from build123d import *

# Parameters (mm, degrees)
BOSS_EXTRUDE1_DEPTH = 10
SKETCH4_W           = 10
SKETCH4_H           = 2.5
SKETCH5_R           = 2.5
BOSS_EXTRUDE2_DEPTH = 5


with BuildPart() as part:
    # Sketch2 → Boss-Extrude1 (new body)
    with BuildSketch(Plane.XY):
        with BuildLine():
            Line((20, 0), (-20, 0))
            ThreePointArc((-20, 0), (0, 20), (20, 0))
        make_face()
    extrude(amount=BOSS_EXTRUDE1_DEPTH)

    # Sketch4 → Cut-Revolve1 (revolve, cut)
    with BuildSketch(Plane(origin=(0, 0, 0), x_dir=(0, 0, -1), z_dir=(1, 0, 0))):
        with Locations((-5, 1.25)):
            Rectangle(SKETCH4_W, SKETCH4_H)
    revolve(axis=Axis((0, 0, 17.133909945), (0, 0, -1)), mode=Mode.SUBTRACT)

    # Sketch5 → Boss-Extrude2 (add)
    with BuildSketch(Plane.XZ):
        with Locations((-15, 5)):
            Circle(SKETCH5_R)
        with Locations((15, 5)):
            Circle(SKETCH5_R)
    extrude(amount=BOSS_EXTRUDE2_DEPTH)


solid = part.part
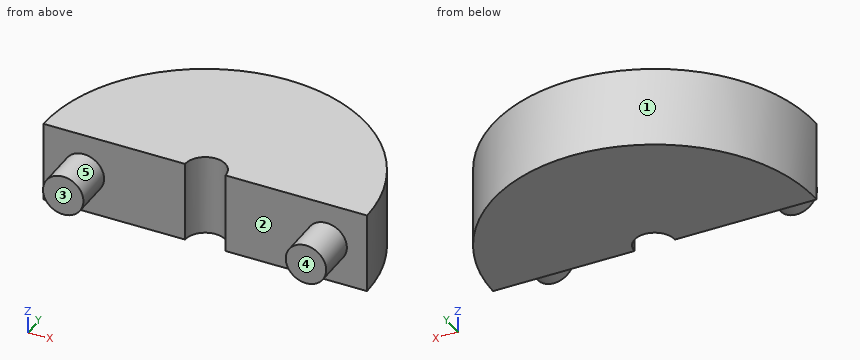
The listing builds one solid part. Answer for the finished solid, in the listing's coordinates (mm). Face numbers are marked on the shaded views. A direction names the side the tool comes from. Coordinates: 2 decimals unless noted, no trailing zeros. Write each loop counter-clockwise with the first axis right and the second up, starting at its lowest first coordinate (ties: lowest second). Pieces come first, ordered by that corner, then holes. Notation, with made-up numbers: (-30, -3) - (-3, -3) arc R6 cw to (-3, 3) - close; hole circle Ø4 at (52, -27). An arc over 180 degrees is marked (long way). Put each result on its own line as item: value.
1. The part is cut by section D-D on z = 5. Give the vertices of the cut face in (x, y).
Answer sheet:
outline: (-20, 0) - (-17.5, 0) - (-17.5, -5) - (-12.5, -5) - (-12.5, 0) - (-2.5, 0) arc R2.5 cw to (2.5, 0) - (12.5, 0) - (12.5, -5) - (17.5, -5) - (17.5, 0) - (20, 0) arc R20 ccw to start
2. The part is cut by section B-B on x = 0. Give the vertices of the cut face in (y, z).
Answer sheet:
outline: (2.5, 0) - (20, 0) - (20, 10) - (2.5, 10) - close
3. The part is cut by section A-A on z = 7. Give the vertices of the cut face in (x, y).
Answer sheet:
outline: (-20, 0) - (-16.5, 0) - (-16.5, -5) - (-13.5, -5) - (-13.5, 0) - (-2.5, 0) arc R2.5 cw to (2.5, 0) - (13.5, 0) - (13.5, -5) - (16.5, -5) - (16.5, 0) - (20, 0) arc R20 ccw to start
4. Flat-ended cylindrical pins translate along their axes: pin 1 Ø1.5 at (x, z) = (-0.5, 9) entering from +Y; pin 2 Ø2 at (y, z) = (11.5, 8.5) entering from -X; pin 3 Ø4 at (x, z) = (1.5, 1.5) entering from -Y. Find the tip coordinate at first contact, or state that the pin passes through.
Answer sheet:
pin 1: stops at y = 20
pin 2: stops at x = -17.02
pin 3: stops at y = 0
5. A tool of negligible diameter and unlimited length cuts with its end or side. For the marked faces 4 and 5, from which of +Z, -Z, +X, -X, +Y, -Y can it reach the whole face along a straight path? Write none if from no direction.
Answer sheet:
face 4: +Z, -Z, +X, -X, -Y
face 5: -Y
6. Find the intervals of material crossed by line 1 along X through (y, z) = (-3.5, 6); line 2 along X through (y, z) = (1.25, 1); line 3 along Y through (x, z) = (4.5, 9), in increasing order. Write a range as from..to.
Answer sheet:
line 1: x = -17.29..-12.71, 12.71..17.29
line 2: x = -19.96..-2.17, 2.17..19.96
line 3: y = 0..19.49
7. The part is cut by section C-C on y = 12. Give the vertices of the cut face in (x, z), plus the area to 3 significant figures.
Answer sheet:
outline: (-16, 0) - (16, 0) - (16, 10) - (-16, 10) - close
area: 320 mm^2
8. Determine the mould class of the marked faces 1, 2 and 3 for opening direction X: pulls with the +X half, pulls with the -X half, needs draft (parallel to the pull), parting line crosses it, or undercut.
Answer sheet:
face 1: parting line crosses it
face 2: undercut
face 3: needs draft
